Geometry: final body of the model. Coordinates: model frame, mm. Give positions to 0.01 mm unless a question says otherwise; leave off trailing zeros. Write each loop counter-clockwise with the first axis right and the second up, starting at its lowest first coordinate (ties: lowest second). Pieces come first, ordered by that corner, then holes. Notation, with made-up numbers: M -36,18.25 L 21,18.25 A23 cw 21,29.25 Z; hole C 73,49.5 d7. An arc over 180 degrees is marked long. Use one line per item in the form item = value. Start each with the question number.
Item 1: Section query A-A on z = -1.5. Give the number of separate pieces and of enclosed holes in the cut face, then the cut area to 3 significant figures.
Item 2: Section query C-C on y = 460. Return loops of the section in (x, z).
Item 3: Contact query for flat-ended pins moving along their axis: P1, Ø0.9, axis at y = 28.5, z = -1, coming from the +X side; P2, Ø0.9, axis at y = 30, z = -1.5, coming from the +X side; P3, Ø1.5, axis at y = 744, z = -1, coming from the +X side. Output: stop coordinate, or through.
Item 4: Material intervals for line 1 along X through (y, z) = (524, -1.95); line 2 along X through (y, z) = (525, -1.8); line 3 along Y through (x, z) = (100, -0.7), sorted ascending. Write a range as from..to.
Item 5: Section query B-B on x = 342.5. Return loops of the section in (y, z).
from build123d import *

# Parameters (mm, degrees)
F0_W     = 143
F0_H     = 20
F1_DEPTH = 3
F2_R     = 2.5
F3_DEPTH = 25
F5_DEPTH = 25
F7_R     = 2.05
F8_DEPTH = 25


with BuildPart() as f1:
    # F0 (on Top) → F1 (new body)
    with BuildSketch(Plane.XY):
        Polygon((0, 1140), (0, 0), (373, 0), (143, 1140), align=None)
        with Locations((71.5, 1150)):
            Rectangle(F0_W, F0_H)
    extrude(amount=-F1_DEPTH)

    # F2 (on face) → F3 (cut)
    with BuildSketch(Plane.XY):
        with Locations((90, 105)):
            Circle(F2_R)
        with Locations((250, 105)):
            Circle(F2_R)
        with Locations((250, 255)):
            Circle(F2_R)
        with Locations((90, 255)):
            Circle(F2_R)
        with Locations((90, 525)):
            Circle(F2_R)
        with Locations((90, 675)):
            Circle(F2_R)
        with Locations((190, 525)):
            Circle(F2_R)
        with Locations((190, 675)):
            Circle(F2_R)
        with Locations((108, 885)):
            Circle(F2_R)
        with Locations((108, 1035)):
            Circle(F2_R)
        with Locations((330, 30)):
            Circle(F2_R)
        with Locations((300, 30)):
            Circle(F2_R)
    extrude(amount=-F3_DEPTH, mode=Mode.SUBTRACT)

    # F4 (on face) → F5 (cut)
    with BuildSketch(Plane.XY):
        with BuildLine():
            ThreePointArc((11.5, 24.5), (15, 21), (18.5, 24.5))
            Line((18.5, 24.5), (18.5, 35.5))
            ThreePointArc((18.5, 35.5), (15, 39), (11.5, 35.5))
            Line((11.5, 35.5), (11.5, 24.5))
        make_face()
        with BuildLine():
            ThreePointArc((41.5, 24.5), (45, 21), (48.5, 24.5))
            Line((48.5, 24.5), (48.5, 35.5))
            ThreePointArc((48.5, 35.5), (45, 39), (41.5, 35.5))
            Line((41.5, 35.5), (41.5, 24.5))
        make_face()
        with BuildLine():
            ThreePointArc((11.5, 574.5), (15, 571), (18.5, 574.5))
            Line((18.5, 574.5), (18.5, 585.5))
            ThreePointArc((18.5, 585.5), (15, 589), (11.5, 585.5))
            Line((11.5, 585.5), (11.5, 574.5))
        make_face()
        with BuildLine():
            ThreePointArc((41.5, 574.5), (45, 571), (48.5, 574.5))
            Line((48.5, 574.5), (48.5, 585.5))
            ThreePointArc((48.5, 585.5), (45, 589), (41.5, 585.5))
            Line((41.5, 585.5), (41.5, 574.5))
        make_face()
        with BuildLine():
            ThreePointArc((11.5, 1124.5), (15, 1121), (18.5, 1124.5))
            Line((18.5, 1124.5), (18.5, 1135.5))
            ThreePointArc((18.5, 1135.5), (15, 1139), (11.5, 1135.5))
            Line((11.5, 1135.5), (11.5, 1124.5))
        make_face()
        with BuildLine():
            ThreePointArc((41.5, 1124.5), (45, 1121), (48.5, 1124.5))
            Line((48.5, 1124.5), (48.5, 1135.5))
            ThreePointArc((48.5, 1135.5), (45, 1139), (41.5, 1135.5))
            Line((41.5, 1135.5), (41.5, 1124.5))
        make_face()
    extrude(amount=-F5_DEPTH, mode=Mode.SUBTRACT)

    # F7 (on face) → F8 (cut)
    with BuildSketch(Plane.XY):
        with Locations((15, 60)):
            Circle(F7_R)
        with Locations((307, 200)):
            Circle(F7_R)
        with Locations((15, 360)):
            Circle(F7_R)
        with Locations((15, 440)):
            Circle(F7_R)
        with Locations((15, 760)):
            Circle(F7_R)
        with Locations((15, 840)):
            Circle(F7_R)
        with Locations((15, 1100)):
            Circle(F7_R)
        with Locations((227, 600)):
            Circle(F7_R)
        with Locations((149, 985)):
            Circle(F7_R)
        with Locations((100, 1100)):
            Circle(F7_R)
        with Locations((140, 1100)):
            Circle(F7_R)
        with Locations((227, 540)):
            Circle(F7_R)
        with Locations((227, 440)):
            Circle(F7_R)
    extrude(amount=-F8_DEPTH, mode=Mode.SUBTRACT)


solid = f1.part
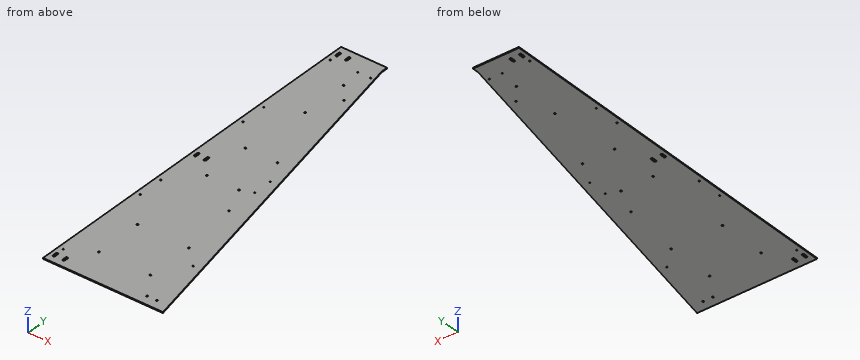
Answer sheet:
q1.separate_pieces = 1
q1.enclosed_holes = 31
q1.area = 296,000 mm2
q2.outline = M 0,-3 L 280.19,-3 L 280.19,0 L 0,0 Z
q3.P1 = 367.34
q3.P2 = 367.04
q3.P3 = 223.05
q4.line_1 = 0..87.71, 92.29..187.71, 192.29..267.28
q4.line_2 = 0..87.5, 92.5..187.5, 192.5..267.08
q4.line_3 = 0..1097.95, 1102.05..1160
q5.outline = M 0,-3 L 151.17,-3 L 151.17,0 L 0,0 Z
